Read the model definition and answer for the solid it produces. Units are mm, in the model's axes. Coordinates: 2 decimals unless noted, no trailing zeros. Write each loop counter-clockwise with the first axis right and the second up, starting at its lowest first coordinate (ties: lowest second). Pieces come first, ordered by that corner, then holes. Notation, with made-up numbers: (-2.5, 0) - (42.5, 0) arc R11 cw to (42.5, 10) - close; hole circle Ø9 at (87.25, 5). An arc over 180 degrees is marked (long way). Use a Markdown table: item, result.
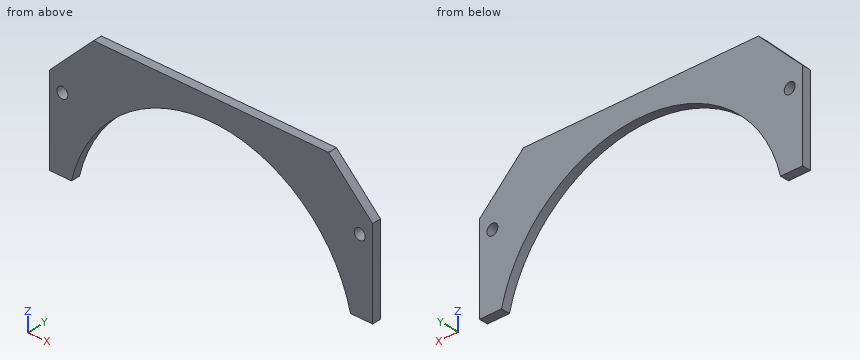
from build123d import *

# Parameters (mm, degrees)
F0_R     = 7.5
F1_DEPTH = 12


with BuildPart() as f1:
    # F0 (on Front) → F1 (new body)
    with BuildSketch(Plane.XZ):
        with BuildLine():
            ThreePointArc((0, 0), (190, 150.027898), (380, 0))
            Line((380, 0), (410, 0))
            Line((410, 0), (410, 120))
            Line((410, 120), (350, 180))
            Line((350, 180), (30, 180))
            Line((30, 180), (-30, 120))
            Line((-30, 120), (-30, 0))
            Line((-30, 0), (0, 0))
        make_face()
        with Locations((-12.5, 100)):
            Circle(F0_R, mode=Mode.SUBTRACT)
        with Locations((392.5, 100)):
            Circle(F0_R, mode=Mode.SUBTRACT)
    extrude(amount=F1_DEPTH)


solid = f1.part
(1) A cutting plane is placed at C-C, the plane z = 100. Write down the section's boundary in (x, y), and give its area (3 significant figures).
Report:
| item | result |
|---|---|
| outline | (-30, -12) - (-20, -12) - (-20, 0) - (-30, 0) - close; (-5, -12) - (59.46, -12) - (59.46, 0) - (-5, 0) - close; (320.54, -12) - (385, -12) - (385, 0) - (320.54, 0) - close; (400, -12) - (410, -12) - (410, 0) - (400, 0) - close |
| area | 1,790 mm² |
(2) A cutting plane is placed at B-B, the plane x = 392.5. Write down the section's boundary in (y, z), and give its area (3 significant figures).
Report:
| item | result |
|---|---|
| outline | (-12, 0) - (0, 0) - (0, 92.5) - (-12, 92.5) - close; (-12, 107.5) - (0, 107.5) - (0, 137.5) - (-12, 137.5) - close |
| area | 1,470 mm² |
(3) A cutting plane is placed at A-A, the plane y = -3. Write down the section's boundary in (x, z).
Report:
| item | result |
|---|---|
| outline | (-30, 0) - (0, 0) arc R195.32 cw to (380, 0) - (410, 0) - (410, 120) - (350, 180) - (30, 180) - (-30, 120) - close; hole circle Ø15 at (-12.5, 100); hole circle Ø15 at (392.5, 100) |
(4) Straight lines are drawn through the part: L1, parallel to Z at x = -12.5, y = -5; L2, parallel to X at y = -5.75, z = 90; L3, parallel to X at y = -7.5, z = 109.5. For each, find the intervals that lie inside material, in ascending order.
Report:
| item | result |
|---|---|
| L1 | z = 0 to 92.5, 107.5 to 137.5 |
| L2 | x = -30 to 49.12, 330.88 to 410 |
| L3 | x = -30 to 70.88, 309.12 to 410 |
(5) A cutting plane is placed at D-D, the plane z = 48.5. Write down the section's boundary in (x, y).
Report:
| item | result |
|---|---|
| outline | (-30, -12) - (18.67, -12) - (18.67, 0) - (-30, 0) - close; (361.33, -12) - (410, -12) - (410, 0) - (361.33, 0) - close |
(6) Each of these flat-tipped pins is pushed along its axis until it touches: P1, Ø1.5, axis at x = 364.5, y = -2, coming from the +Z side; P2, Ø9, axis at x = 392.5, z = 100, coming from the +Y side; P3, Ø4, axis at x = 291.5, y = -2.5, coming from the -Z side. Where does it stop, or does it pass through?
Report:
| item | result |
|---|---|
| P1 | stops at z = 166.25 |
| P2 | passes through |
| P3 | stops at z = 120.35 |
